Study the drawing (mm; zero at the part's minimum x, y, z) and answer. Coordinates: 2 decimals unless noted, no trailing zeros. Loops run counter-clockwise (first coordinate to the right, second up) from the corner with the lowest first, then second, coordinate; pieces in that order, holes last. Notation, with made-up numbers: (89, 37) -> (143, 37) arc R23 ccw to (143, 69) -> close; hole circle Ø3 at (36.25, 57.5). An arc over 180 degrees is marked (long way). Answer in a Markdown table with one row per item.
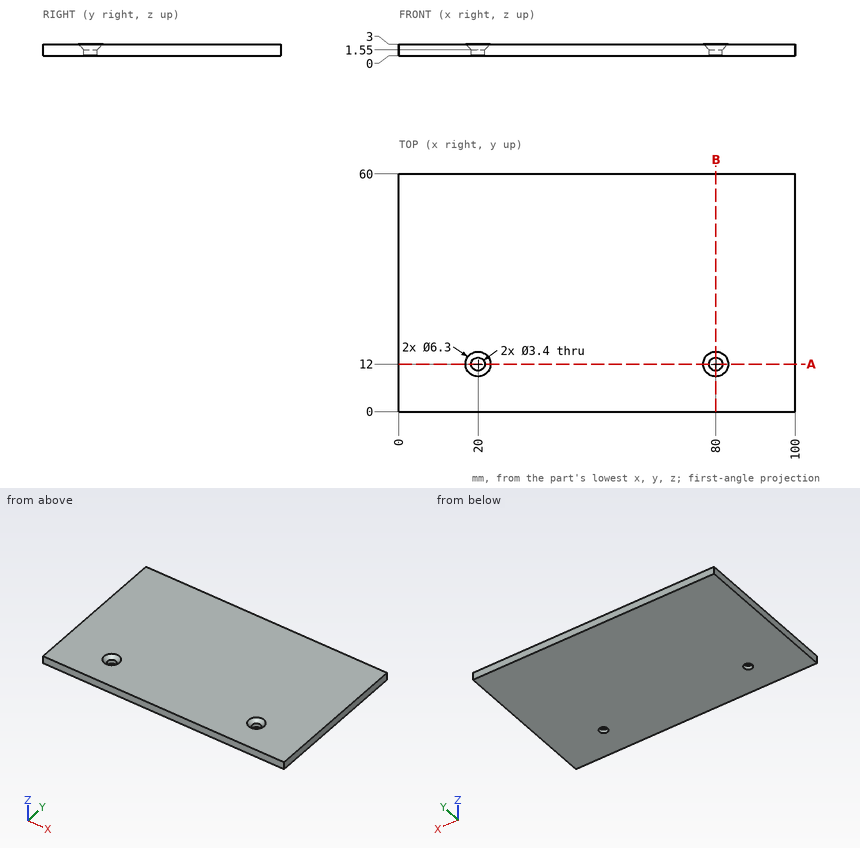
1. A cutting plane is placed at B-B on x = 80. Give the vertices of the cut face in (y, z).
A:
| item | result |
|---|---|
| outline | (0, 0) -> (10.3, 0) -> (10.3, 1.55) -> (8.85, 3) -> (0, 3) -> close; (13.7, 0) -> (60, 0) -> (60, 3) -> (15.15, 3) -> (13.7, 1.55) -> close |
2. A cutting plane is placed at A-A on y = 12. Give the vertices of the cut face in (x, z).
A:
| item | result |
|---|---|
| outline | (0, 0) -> (18.3, 0) -> (18.3, 1.55) -> (16.85, 3) -> (0, 3) -> close; (21.7, 0) -> (78.3, 0) -> (78.3, 1.55) -> (76.85, 3) -> (23.15, 3) -> (21.7, 1.55) -> close; (81.7, 0) -> (100, 0) -> (100, 3) -> (83.15, 3) -> (81.7, 1.55) -> close |
3. Given pin 1 Ø2.5 at (x, y) = (20, 12) entering from -Z, flat-ended and moving along its own axis, determine where the tip first touches the part or whether it passes through.
A:
| item | result |
|---|---|
| pin 1 | passes through |
4. Find the intervals of material crossed by probe 1 along X at (y, z) = (12, 0.4); probe 2 along Y at (x, z) = (20, 1.2); probe 3 along Y at (x, z) = (79, 1.65), in increasing order.
A:
| item | result |
|---|---|
| probe 1 | x = 0 to 18.3, 21.7 to 78.3, 81.7 to 100 |
| probe 2 | y = 0 to 10.3, 13.7 to 60 |
| probe 3 | y = 0 to 10.5, 13.5 to 60 |
